Check sheet for the modelled part. Datum: model origin and axes. Units: mm. A direction names the side the tool comes from. Give positions to 0.01 mm unless a question says otherwise; leave off trailing zeros. Loops run counter-clockwise (first coordinate to the right, second up) from the corner with the lowest first, then second, coordinate; pieces in that order, holes last. Notation, with made-up numbers: (89.5, -8.5) -> (128.5, -8.5) arc R14 ccw to (128.5, -3.5) -> close; hole circle Ø4 at (23, 76). An arc over 180 degrees is marked (long way). Write each question's results on one line, items separated by ' | '. Start each with the question number.
1. Tool access check on faces 1 (the face through (-73.75, 279.07, 55.46)), 2 (the face through (-54.93, 202, 55.91)), 3 (the face through (-31, 271, 56.962)), 4 (the face through (-80, 234, 5)), 5 (the face through (-73.457, 233.665, 24.844)). Record the directions out of +Z, -Z, +X, -X, +Y, -Y that give a thin tool (end or side, any length) a straight path to the whole face; none if there is none.
2. Cross-section at B-B on x = -5. Record the boundary of the cut face in (y, z).
3. Mould release check, pull along Z, two halves, no side actions. Record for faces 6 (the face through (-54, 234, 5)), 7 (the face through (-92.75, 186.93, 55.46)): +Z half, -Z half, draft (parallel to the pull), parting line (faces both ways), or undercut.
4. Gauge pin test, flat ends, axial feed: pin 1 Ø13 at (x, y) = (-53.5, 233.5) entering from +Z; pin 2 Ø1.5 at (y, z) = (245.5, 3) entering from -X; pin 3 Ø1 at (y, z) = (196.5, 10.5) entering from -X. Record the tip position at first contact, or that the pin passes through.
5. Cross-section at A-A on z = 28.5. Record the boundary of the cut face in (x, y), and give its area (4 significant figures).
6. Cross-section at D-D on z = 37. Count the separate pieces of the cut face and the enclosed holes in it, and give its area (3 significant figures).
7. Material ranges on L1, parallel to Z at x = -30.5, y = 270.5; L2, parallel to X at y = 197, z = 30.5; L3, parallel to X at y = 270, z = 44.5, recorded low to high. Write a range as from..to.
8. Cross-section at C-C on y = 225. Record the boundary of the cut face in (x, z).
from build123d import *

# Parameters (mm, degrees)
SKETCH026_W     = 95
SKETCH026_H     = 95
PAD018_DEPTH    = 5
PAD019_DEPTH    = 95
SKETCH028_R     = 30
POCKET008_DEPTH = 95.501
FILLET020_R     = 5
FILLET021_R     = 2


with BuildPart() as part:
    # Sketch026 → Pad018 (new body)
    with BuildSketch(Plane.XY):
        Rectangle(SKETCH026_W, SKETCH026_H)
    extrude(amount=PAD018_DEPTH)

    # Sketch027 (on DatumPlane) → Pad019 (join)
    with BuildSketch(Plane(origin=(0, 47.5, 0), x_dir=(-1, 0, 0), z_dir=(0, 1, 0))):
        Polygon((-47, 5), (-17, 56.961524), (-14, 56.961524), (-44, 5), align=None)
        Polygon((-37, 5), (-7, 56.961524), (-4, 56.961524), (-34, 5), align=None)
        Polygon((-23, 5), (7, 56.961524), (10, 56.961524), (-20, 5), align=None)
        Polygon((-4, 5), (26, 56.961524), (29, 56.961524), (-1, 5), align=None)
        Polygon((15, 5), (45, 56.961524), (48, 56.961524), (18, 5), align=None)
    extrude(amount=-PAD019_DEPTH)

    # Sketch028 (on DatumPlane) → Pocket008 (cut, through all)
    with BuildSketch(Plane.YZ.offset(47.5)):
        with Locations((0, 60)):
            Circle(SKETCH028_R)
    extrude(amount=-POCKET008_DEPTH, mode=Mode.SUBTRACT)

    # Fillet020
    fillet020_edges = [part.edges().sort_by_distance(p)[0] for p in [
        (15.5, -47.5, 56.961524),
        (15.5, -29.845731, 56.961524),
        (5.5, -47.5, 56.961524),
        (5.5, -29.845731, 56.961524),
        (-8.5, -47.5, 56.961524),
        (-8.5, -29.845731, 56.961524),
        (-27.5, -47.5, 56.961524),
        (-27.5, -29.845731, 56.961524),
        (-46.5, -47.5, 56.961524),
        (-46.5, -29.845731, 56.961524),
        (15.5, 29.845731, 56.961524),
        (15.5, 47.5, 56.961524),
        (5.5, 29.845731, 56.961524),
        (5.5, 47.5, 56.961524),
        (-8.5, 29.845731, 56.961524),
        (-8.5, 47.5, 56.961524),
        (-27.5, 29.845731, 56.961524),
        (-27.5, 47.5, 56.961524),
        (-46.5, 29.845731, 56.961524),
        (-46.5, 47.5, 56.961524),
    ]]
    fillet(fillet020_edges, radius=FILLET020_R)

    # Fillet021
    fillet021_edges = [part.edges().sort_by_distance(p)[0] for p in [
        (0, 47.5, 0),
        (47.5, 0, 0),
        (0, -47.5, 0),
        (-47.5, 0, 0),
    ]]
    fillet(fillet021_edges, radius=FILLET021_R)


with BuildPart() as part_1:
    # Body012 placement: moved
    add(part.part.moved(Location((-47, 233, 0))))


solid = part_1.part
Geometry says:
1) face 1: +Z, +X, -X, +Y | face 2: +Z, +X, -X | face 3: +Z, +X, -X, +Y, -Y | face 4: -X, +Y, -Y | face 5: +Y, -Y
2) outline: (185.5, 2) arc R2 ccw to (187.5, 0) -> (278.5, 0) arc R2 ccw to (280.5, 2) -> (280.5, 5) -> (185.5, 5) -> close; (185.5, 8.46) -> (280.5, 8.46) -> (280.5, 13.66) -> (185.5, 13.66) -> close
3) face 6: undercut | face 7: +Z half
4) pin 1: z = 30.5 | pin 2: x = -94.5 | pin 3: x = -68.46
5) outline: (-78.57, 185.5) -> (-75.57, 185.5) -> (-75.57, 280.5) -> (-78.57, 280.5) -> close; (-59.57, 185.5) -> (-56.57, 185.5) -> (-56.57, 280.5) -> (-59.57, 280.5) -> close; (-40.57, 185.5) -> (-37.57, 185.5) -> (-37.57, 280.5) -> (-40.57, 280.5) -> close; (-26.57, 185.5) -> (-23.57, 185.5) -> (-23.57, 280.5) -> (-26.57, 280.5) -> close; (-16.57, 185.5) -> (-13.57, 185.5) -> (-13.57, 280.5) -> (-16.57, 280.5) -> close | area: 1,425 mm^2
6) separate pieces: 10 | enclosed holes: 0 | area: 847 mm^2
7) L1: 0..5, 11.06..16.26, 35.31..40.51, 52.63..56.96 | L2: -79.72..-76.72, -60.72..-57.72, -41.72..-38.72, -27.72..-24.72, -17.72..-14.72 | L3: -87.81..-84.81, -68.81..-65.81, -49.81..-46.81, -35.81..-32.81, -25.81..-22.81
8) outline: (-94.5, 2) arc R2 ccw to (-92.5, 0) -> (-1.5, 0) arc R2 ccw to (0.5, 2) -> (0.5, 5) -> (0, 5) -> (-15.06, 31.09) -> (-18.06, 31.09) -> (-3, 5) -> (-10, 5) -> (-25.06, 31.09) -> (-28.06, 31.09) -> (-13, 5) -> (-24, 5) -> (-39.06, 31.09) -> (-42.06, 31.09) -> (-27, 5) -> (-43, 5) -> (-58.06, 31.09) -> (-61.06, 31.09) -> (-46, 5) -> (-62, 5) -> (-77.06, 31.09) -> (-80.06, 31.09) -> (-65, 5) -> (-94.5, 5) -> close
